The listing builds one solid part. Answer for the finished solid, in the listing's coordinates (mm). A direction names the side the tool comes from. Give positions to 0.01 mm unless a question says otherwise; leave off trailing zeros. Loops run counter-clockwise (first coordinate to the right, second up) from the corner with the lowest first, then second, coordinate; pieces in that order, holes last. Notation, with made-up numbers: (63, 13.25) - (112, 13.25) arc R21 cw to (112, 45.25) - close; hole circle Ø2 at (33, 71.25). An arc over 180 degrees is marked (long way). Answer as CSV lines item,"result". Start each with the question number.
1) Find the intervals of material crossed by line 1 along Z through (x, y) = (37, -1); line 2 along Z through (x, y) = (-2.55, 19) (3 decimals); line 3 along Z through (x, y) = (21.5, -1.25), in increasing order.
2) Flat-ended cylindrical pins translate along their axes: pin 1 (9 mm diameter, centred on y = 19, z = 55, fed in from +X); pin 2 (4.5 mm diameter, centred on x = -3.5, z = 61, fed in from -Y); pin 3 (9 mm diameter, centred on y = 20, z = 76.5, fed in from +X); pin 4 (15 mm diameter, centred on x = 21.5, z = 21.5, fed in from -Y). Find the tip coordinate at first contact, or state that the pin passes through.
3) A cutting plane is placed at B-B (x = 6). Determine the outline of the cut face in (y, z).
4) A cutting plane is placed at D-D (x = 37). Determine the outline of the cut face in (y, z), and give its area (3 significant figures).
5) For faces 4 (the face through (-1, 20, 66)), 5 (the face through (-3, 19, 51)), 6 (the face through (-3, 55, 30)), 7 (the face through (-1, 27, 22)), 8 (the face through (-3, 5, 64)), determine the directions among +Z, -Z, +X, -X, +Y, -Y from which every point of the face is accessible in a straight line to the end or side of a thin tool.
6) A cutting plane is placed at C-C (y = 19.5). Determine the outline of the cut face in (x, z).
7) For a pull along Y with two mould halves and no side action, classify faces 1 (the face through (-3, 34, 62)), 2 (the face through (-1.986, 18.268, 80.577)), 3 (the face through (-5, 25, 35)) as pulls with the +Y half, pulls with the -Y half, needs draft (parallel to the pull), parting line crosses it, or undercut.
8) A cutting plane is placed at A-A (z = 37). Determine the outline of the cut face in (x, y).
```python
from build123d import *

# Parameters (mm, degrees)
F1_W           = 48
F1_H           = 47
F2_DEPTH       = 2.5
F4_DEPTH       = 4
F6_DEPTH       = 3
F8_D           = 6.6
F8_CBORE_D     = 11.25
F8_CBORE_DEPTH = 2
F9_R           = 1.5
F9_R_2         = 12.5
F10_DEPTH      = 2.501
F11_SIZE       = 1.5


with BuildPart() as f2:
    # F1 (on Front) → F2 (new body)
    with BuildSketch(Plane.XZ):
        with Locations((19, 23.5)):
            Rectangle(F1_W, F1_H)
    extrude(amount=F2_DEPTH)

    # F3 (on face) → F4 (join)
    with BuildSketch(Plane(origin=(-5, 0, 0), x_dir=(0, -1, 0), z_dir=(-1, 0, 0))):
        Polygon((-62.5, 0), (0, 0), (0, 47), (-5, 47), (-5, 80.5), (-9.5, 85), (-29.5, 85), (-34, 80.5), (-34, 43.5), (-47.5, 30), (-62.5, 30), (-67.5, 25), (-67.5, 5), align=None)
    extrude(amount=-F4_DEPTH)

    # F5 (on face) → F6 (join)
    with BuildSketch(Plane.XY.offset(47)):
        Polygon((-1, 5), (-1, 0), (43, 0), (-1, 34), align=None)
    extrude(amount=-F6_DEPTH)

    # F8 (through all)
    with Locations(Plane.YZ.offset(-1)):
        with Locations((19, 75), (19, 55), (57.5, 15)):
            CounterBoreHole(F8_D / 2, F8_CBORE_D / 2, F8_CBORE_DEPTH)

    # F9 (on face) → F10 (cut, through all)
    with BuildSketch(Plane(origin=(0, 0, 0), x_dir=(-1, 0, 0), z_dir=(0, 1, 0))):
        with Locations((-37, 37)):
            Circle(F9_R)
        with Locations((-37, 6)):
            Circle(F9_R)
        with Locations((-6, 6)):
            Circle(F9_R)
        with Locations((-21.5, 21.5)):
            Circle(F9_R_2)
    extrude(amount=-F10_DEPTH, mode=Mode.SUBTRACT)

    # F11
    f11_edges = [f2.edges().sort_by_distance(p)[0] for p in [
        (43, -1.25, 0),
        (-5, 30, 0),
    ]]
    chamfer(f11_edges, length=F11_SIZE)


solid = f2.part
```
Ans:
1,line 1,"0 to 4.5, 7.5 to 35.5, 38.5 to 47"
1,line 2,"0 to 49.375, 60.625 to 69.375, 80.625 to 85"
1,line 3,"0 to 9, 34 to 47"
2,pin 1,"x = -3"
2,pin 2,"y = 5"
2,pin 3,"x = -1"
2,pin 4,"through"
3,outline,"(-2.5, 0) - (0, 0) - (0, 4.5) - (-2.5, 4.5) - close; (-2.5, 7.5) - (0, 7.5) - (0, 44) - (28.59, 44) - (28.59, 47) - (-2.5, 47) - close"
4,outline,"(-2.5, 0) - (0, 0) - (0, 4.5) - (-2.5, 4.5) - close; (-2.5, 7.5) - (0, 7.5) - (0, 35.5) - (-2.5, 35.5) - close; (-2.5, 38.5) - (0, 38.5) - (0, 44) - (4.64, 44) - (4.64, 47) - (-2.5, 47) - close"
4,area,"116 mm2"
5,face 4,"+Z, +X, +Y, -Y"
5,face 5,"+X"
5,face 6,"+Z, +X, -X, +Y"
5,face 7,"-Z, +X, +Y"
5,face 8,"+Z, +X, -X, -Y"
6,outline,"(-5, 1.5) - (-3.5, 0) - (-1, 0) - (-1, 44) - (17.76, 44) - (17.76, 47) - (-1, 47) - (-1, 49.4) - (-3, 49.4) - (-3, 51.74) - (-5, 51.74) - close; (-5, 58.26) - (-3, 58.26) - (-3, 60.6) - (-1, 60.6) - (-1, 69.4) - (-3, 69.4) - (-3, 71.74) - (-5, 71.74) - close; (-5, 78.26) - (-3, 78.26) - (-3, 80.6) - (-1, 80.6) - (-1, 85) - (-5, 85) - close"
7,face 1,"pulls with the +Y half"
7,face 2,"undercut"
7,face 3,"needs draft"
8,outline,"(-5, -2.5) - (35.5, -2.5) - (35.5, 0) - (-1, 0) - (-1, 40.5) - (-5, 40.5) - close; (38.5, -2.5) - (43, -2.5) - (43, 0) - (38.5, 0) - close"
